Input: part model. Units: mm. Frame: model coordinates. Round coordinates to 2 decimals unless told otherwise and drop trailing zeros. Order: outer loops, then holes, each group sorted by start corner. A loop starts at its lowest first (then second) coordinate and runs counter-clockwise, first axis right, second up. Notation, with made-up numbers: M -15.75,-27 L 13.25,-27 A18 cw 13.25,-2 Z; hole C 6,-13.75 d11. An arc over 180 degrees is marked long. One line per question, with ' | ' between items.
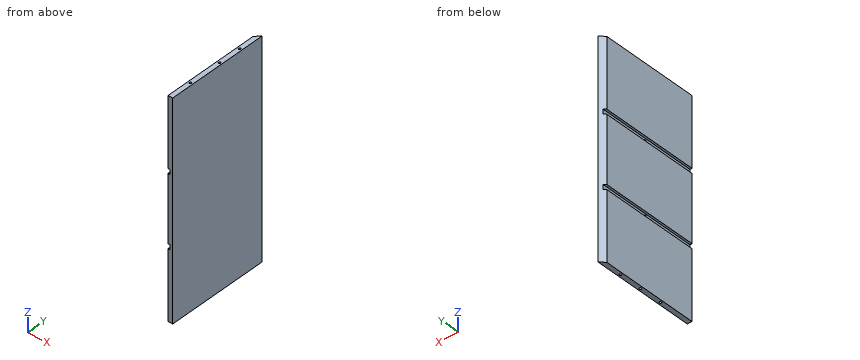
```python
from build123d import *

# Parameters (mm, degrees)
F0_W           = 390
F0_H           = 260
F0_H_2         = 251
F0_H_3         = 18
F1_DEPTH       = 18
F2_DEPTH       = 8
F3_SIZE2       = 17.99999
F3_SIZE        = 17.99999
F6_D           = 8
F6_DEPTH       = 21
F6_TIP         = 2.4034424761
F6_ON_F5_D     = 8
F6_ON_F5_DEPTH = 21
F6_ON_F5_TIP   = 2.4034424761
F8_D           = 8
F8_DEPTH       = 11
F8_TIP         = 2.4034424761


# Not quite as in the source:
# - a fillet or chamfer is up to 0.001 mm smaller than in the source, because OpenCascade refuses the exact size


with BuildPart() as f1:
    # F0 (on Right) → F1 (new body)
    with BuildSketch(Plane.YZ):
        with Locations((0, 273.5)):
            Rectangle(F0_W, F0_H)
        Rectangle(F0_W, F0_H_2)
        with Locations((0, -273.5)):
            Rectangle(F0_W, F0_H)
        with Locations((0, 134.5)):
            Rectangle(F0_W, F0_H_3)
        with Locations((0, -134.5)):
            Rectangle(F0_W, F0_H_3)
    extrude(amount=F1_DEPTH)

    # F0 (on Right) → F2 (cut)
    with BuildSketch(Plane.YZ):
        with Locations((0, 134.5)):
            Rectangle(F0_W, F0_H_3)
        with Locations((0, -134.5)):
            Rectangle(F0_W, F0_H_3)
    extrude(amount=F2_DEPTH, mode=Mode.SUBTRACT)

    # F3 (size 18 and 18 in the source; OpenCascade refuses exactly that, so slightly less here)
    f3_edges = [f1.edges().sort_by_distance(p)[0] for p in [
        (0, 195, 0),
    ]]
    chamfer(f3_edges, length=F3_SIZE, length2=F3_SIZE2)

    # F6
    with Locations(Plane.XY.offset(403.5)):
        with Locations((9, 107.5), (9, 20), (9, -107.5)):
            Hole(F6_D / 2, depth=F6_DEPTH)
            with Locations((0, 0, -(F6_DEPTH + F6_TIP / 2))):  # 118° drill point
                Cone(0, F6_D / 2, F6_TIP, mode=Mode.SUBTRACT)

    # F6 on F5
    with Locations(Plane(origin=(0, 0, -403.5), x_dir=(1, 0, 0), z_dir=(0, 0, -1))):
        with Locations((9, -107.5), (9, -20), (9, 67.5)):
            Hole(F6_ON_F5_D / 2, depth=F6_ON_F5_DEPTH)
            with Locations((0, 0, -(F6_ON_F5_DEPTH + F6_ON_F5_TIP / 2))):  # 118° drill point
                Cone(0, F6_ON_F5_D / 2, F6_ON_F5_TIP, mode=Mode.SUBTRACT)

    # F8
    with Locations(Plane(origin=(0, 0, 0), x_dir=(0, 1, 0), z_dir=(-1, 0, 0))):
        with Locations((0, 134.5), (0, -134.5)):
            Hole(F8_D / 2, depth=F8_DEPTH)
            with Locations((0, 0, -(F8_DEPTH + F8_TIP / 2))):  # 118° drill point
                Cone(0, F8_D / 2, F8_TIP, mode=Mode.SUBTRACT)


solid = f1.part
```
Item 1: Line query: line 1 along Z through (x, y) = (5, 34); line 2 along Y through (x, z) = (9, -392.5); line 3 along Y through (x, z) = (9, 392.25). Output: solid intervals per line, ascending. Write a range as from..to.
Report:
line 1: -403.5..-143.5, -125.5..125.5, 143.5..403.5 | line 2: -195..-71.5, -63.5..16, 24..103.5, 111.5..186 | line 3: -195..-111.5, -103.5..16, 24..103.5, 111.5..186
Item 2: Section query B-B, the plane y = 75. Return loops of the section in (x, z), plus the area to 3 significant figures.
Report:
outline: M 0,-403.5 L 18,-403.5 L 18,403.5 L 0,403.5 L 0,143.5 L 8,143.5 L 8,125.5 L 0,125.5 L 0,-125.5 L 8,-125.5 L 8,-143.5 L 0,-143.5 Z | area: 14,200 mm²
Item 3: First-contact query: pin 1 (5 mm diameter, centred on x = 9, y = 20, fed in from +Z); pin 2 (9 mm diameter, centred on y = 51, z = -133.5, fed in from -X); pin 3 (7 mm diameter, centred on x = 9, y = 20, fed in from -Z); pin 4 (20 mm diameter, centred on y = -42.5, z = 138.5, fed in from -X). Flat tips, straight axial feed; report the tip coordinate or a pass-through.
Report:
pin 1: z = 381.6 | pin 2: x = 8 | pin 3: z = -382.2 | pin 4: x = 0
